The drawing under review shows one solid part. Ordinate dimensions are in mm from its lowest x, y, z. Coordinates: 2 decimals unless noted, no trailing zeros. Write each loop counter-clockwise with the first axis right and the second up, starting at its lowest first coordinate (ties: lowest second). Pieces come first, ordered by that corner, then holes.
1) Add section B-B, the plane x = 102. State the section outline as (y, z) points (1 decimal), then the cut area to 3 significant figures.
2) Add section C-C, the plane y = 8. Give the number of separate pieces and of enclosed holes in the cut face, then the cut area to 3 significant figures.
3) For P1, Ø2.5, axis at x = 184.09, z = 49.5, coming from the +Y side; P2, Ø5, axis at y = 6.5, z = 123.5, coming from the +X side; P3, Ø4, axis at y = 8, z = 30, coming from the -X side, all flat-tipped, find the tip position at first contact; note any pin that passes through.
4) Add section A-A, the plane z = 120. State the section outline as (x, y) points (1 decimal).
5) For line 1 (X direction, y = 6.75, z = 28.5) (1 decimal), list the stretches that pass through material, from the lowest coordinate up.
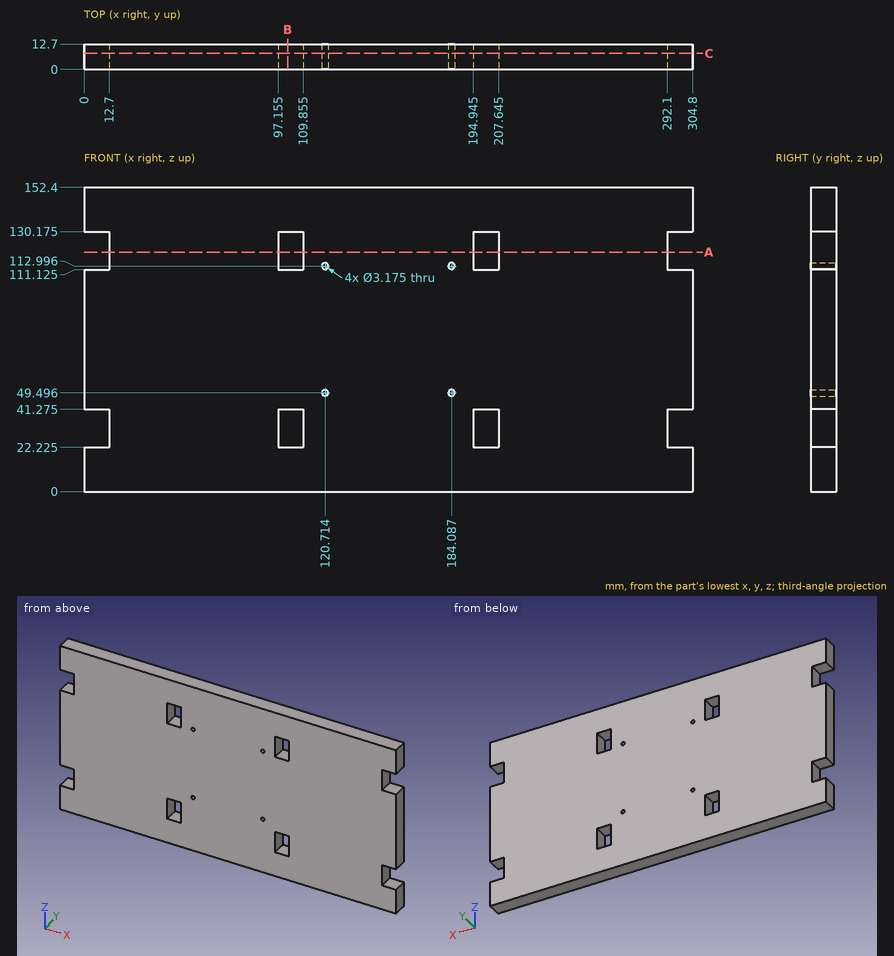
Geometry results:
1. outline: (0, 0) - (12.7, 0) - (12.7, 22.2) - (0, 22.2) - close; (0, 41.3) - (12.7, 41.3) - (12.7, 111.1) - (0, 111.1) - close; (0, 130.2) - (12.7, 130.2) - (12.7, 152.4) - (0, 152.4) - close
1. area: 1,450 mm2
2. separate pieces: 1
2. enclosed holes: 8
2. area: 44,500 mm2
3. P1: passes through
3. P2: stops at x = 292.1
3. P3: stops at x = 12.7
4. outline: (12.7, 0) - (97.2, 0) - (97.2, 12.7) - (12.7, 12.7) - close; (109.9, 0) - (194.9, 0) - (194.9, 12.7) - (109.9, 12.7) - close; (207.6, 0) - (292.1, 0) - (292.1, 12.7) - (207.6, 12.7) - close
5. line 1: x = 12.7 to 97.2, 109.9 to 194.9, 207.6 to 292.1
